The model under review builds one solid part; all positions refer to its coordinate system, in mm. Face numbers are marked on the shaded views. Round coordinates to 2 decimals unless told otherwise and drop trailing zeros. Order: outer loops, then holes, each group sorted by start corner. A loop starts at its lowest first (then second) coordinate and runs counter-clockwise, first axis right, second up. Notation, with made-up numbers: (-16, -1) -> (2, -1) arc R27 ccw to (2, 32) -> close; hole circle Ø5 at (74.25, 6). An arc over 180 degrees is marked (long way). Return JSON: item names as keys, results as strings. Group by question number.
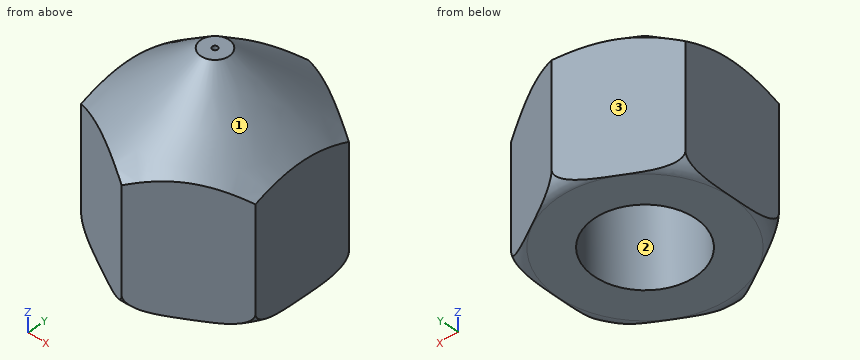
from build123d import *

# Parameters (mm, degrees)
SKETCH_1_R          = 6.466323015
EXTRUDE_1_DEPTH     = 7.5
SKETCH_2_R          = 6.466323015
EXTRUDE_2_DEPTH     = 4.5
EXTRUDE_2_TAPER     = 51
FILLET_1_R          = 0.9
SKETCH_3_OUTSIDE_W  = 19.306
SKETCH_3_OUTSIDE_H  = 19.306
CUT_EXTRUDE_2_DEPTH = 16.087301504
SKETCH_4_R          = 3.25
CUT_EXTRUDE_3_DEPTH = 8
SKETCH_6_R          = 0.175
CUT_EXTRUDE_4_DEPTH = 15.736802168
SKETCH_5_R          = 1.09
CUT_EXTRUDE_5_DEPTH = 3.5
CUT_EXTRUDE_5_DRAFT = -15


with BuildPart() as part:
    # Эскиз1 → Бобышка-Вытянуть1 (new body)
    with BuildSketch(Plane.XY):
        Circle(SKETCH_1_R)
    extrude(amount=EXTRUDE_1_DEPTH)

    # Эскиз2 → Бобышка-Вытянуть2 (add)
    with BuildSketch(Plane.XY.offset(7.5)):
        Circle(SKETCH_2_R)
    extrude(amount=EXTRUDE_2_DEPTH, taper=EXTRUDE_2_TAPER)

    # Скругление1
    fillet_1_edges = [part.edges().sort_by_distance(p)[0] for p in [
        (-6.466323015, 0, 0),
    ]]
    fillet(fillet_1_edges, radius=FILLET_1_R)

    # Эскиз3 outside → Вырез-Вытянуть2 (cut, through all)
    with BuildSketch(Plane(origin=(0, 0, 0), x_dir=(-1, 0, 0), z_dir=(0, 0, -1))):
        Rectangle(SKETCH_3_OUTSIDE_W, SKETCH_3_OUTSIDE_H)
        Polygon((0, 6.466323015), (-5.6, 3.233161507), (-5.6, -3.233161507), (0, -6.466323015), (5.6, -3.233161507), (5.6, 3.233161507), align=None, mode=Mode.SUBTRACT)
    extrude(amount=-CUT_EXTRUDE_2_DEPTH, mode=Mode.SUBTRACT)

    # Эскиз4 → Вырез-Вытянуть3 (cut)
    with BuildSketch(Plane(origin=(0, 0, 0), x_dir=(-1, 0, 0), z_dir=(0, 0, -1))):
        Circle(SKETCH_4_R)
    extrude(amount=-CUT_EXTRUDE_3_DEPTH, mode=Mode.SUBTRACT)

    # Эскиз6 → Вырез-Вытянуть4 (cut, through all)
    with BuildSketch(Plane.XY.offset(12)):
        Circle(SKETCH_6_R)
    extrude(amount=-CUT_EXTRUDE_4_DEPTH, mode=Mode.SUBTRACT)


with BuildPart() as cut_extrude_5_tool:
    # Эскиз5 → Вырез-Вытянуть5 (with draft: the straight prism first)
    with BuildSketch(Plane(origin=(0, 0, 8), x_dir=(-1, 0, 0), z_dir=(0, 0, -1))):
        Circle(SKETCH_5_R)
    extrude(amount=-CUT_EXTRUDE_5_DEPTH)
    # Вырез-Вытянуть5: the draft: its side faces are tilted about the plane it starts from
    cut_extrude_5_sides = [cut_extrude_5_tool.faces().sort_by_distance(p)[0] for p in [
        (1.09, 0, 9.75),
    ]]
    draft(cut_extrude_5_sides, Plane(origin=(0, 0, 8), x_dir=(-1, 0, 0), z_dir=(0, 0, -1)), CUT_EXTRUDE_5_DRAFT)


with BuildPart() as part_1:
    add(part.part)

    # Вырез-Вытянуть5: cut by cut_extrude_5_tool
    add(cut_extrude_5_tool.part, mode=Mode.SUBTRACT)


solid = part_1.part
Item 1: Consider section A-A on y = 0. State the section outline as (x, z) points (3 decimals).
Item 2: Wall thickness on line 1 along X through (y, z) = (0, 11.7) (3 decimals); line 2 along Y through (x, z) = (0.5, 6.25); line 3 along X through (y, z) = (-0.5, 4.5): over which ranges is each line inside the solid? List them lowest first.
Item 3: The part is to be moulded in two halves that separate along X. For the marked faces 1, 2 and 3, say which applies: +X half, -X half, draft (parallel to the pull), parting line (faces both ways), or undercut.
Item 4: Consider section B-B on z = 6.5. State the section outline as (x, y) points.
Item 5: Insertion check: pin 1 Ø1.5 at (y, z) = (4.5, 8) entering from +X; pin 2 Ø1 at (x, z) = (-3, 7) entering from +Y; pin 3 Ø3 at (x, z) = (-3.5, 3.5) entering from +Y. Each pin has a flat end and moves straight along its axis. Give the tip position at first contact, or say it passes through.
Values:
{
 "1": {"outline": "(-5.6, 0.001) arc R0.9 ccw to (-5.566, 0) -> (-3.25, 0) -> (-3.25, 8) -> (-1.09, 8) -> (-0.175, 11.415) -> (-0.175, 12) -> (-0.909, 12) -> (-5.6, 8.202) -> close; (0.175, 11.415) -> (1.09, 8) -> (3.25, 8) -> (3.25, 0) -> (5.566, 0) arc R0.9 ccw to (5.6, 0.001) -> (5.6, 8.202) -> (0.909, 12) -> (0.175, 12) -> close"},
 "2": {"line 1": "-1.28 to -0.175, 0.175 to 1.28", "line 2": "-6.18 to -3.21, 3.21 to 6.18", "line 3": "-5.6 to -3.21, 3.21 to 5.6"},
 "3": {"face 1": "parting line", "face 2": "undercut", "face 3": "-X half"},
 "4": {"outline": "(-5.6, -3.23) -> (0, -6.47) -> (5.6, -3.23) -> (5.6, 3.23) -> (0, 6.47) -> (-5.6, 3.23) -> close; hole circle Ø6.5 at (0, 0)"},
 "5": {"pin 1": "x = 4.69", "pin 2": "y = 5.02", "pin 3": "y = 5.31"}
}
